Model file for the job. Use its own axes, mm. A direction names the side the tool comes from. Coordinates: 2 decimals unless noted, no trailing zeros. Loops run counter-clockwise (first coordinate to the right, second up) from the corner with the lowest first, then second, coordinate; pieces in that order, holes last. Notation, with made-up numbers: (68, 79) -> (83, 79) arc R12 cw to (83, 95) -> close; hole circle Ø2 at (-37.5, -31.5). An arc over 180 degrees is marked (long way). Use one line per item in the form item = value.
```python
from build123d import *

# Parameters (mm, degrees)
SKETCH1_W           = 150
SKETCH1_H           = 40
BOSS_EXTRUDE1_DEPTH = 10
BOSS_EXTRUDE2_DEPTH = 10
CUT_EXTRUDE1_DEPTH  = 121.208152802
SKETCH8_R           = 3.5
CUT_EXTRUDE2_DEPTH  = 108.935165725
FILLET1_R           = 3


with BuildPart() as part:
    # Sketch1 → Boss-Extrude1 (new body)
    with BuildSketch(Plane(origin=(0, 0, 0), x_dir=(1, 0, 0), z_dir=(0, 1, 0))):
        Rectangle(SKETCH1_W, SKETCH1_H)
    extrude(amount=BOSS_EXTRUDE1_DEPTH)

    # Sketch2 → Boss-Extrude2 (add)
    with BuildSketch(Plane.XY.offset(20)):
        with BuildLine():
            Line((-45, 10), (-5, 10))
            Line((-5, 10), (-5, 65))
            ThreePointArc((-5, 65), (-25, 85), (-45, 65))
            Line((-45, 65), (-45, 10))
        make_face()
    extrude(amount=-BOSS_EXTRUDE2_DEPTH)

    # Sketch6 → CBORE for M6 SBHCS1 (revolve, cut)
    with BuildSketch(Plane(origin=(-25, 65, 10), x_dir=(0, 1, 0), z_dir=(1, 0, 0))):
        Polygon((0, 0), (0, 10), (9.005, 10), (9.005, 5.68), (4.5, 5.68), (4.5, 0), align=None)
    revolve(axis=Axis((-25, 65, 3.65), (0, 0, 1)), mode=Mode.SUBTRACT)

    # Sketch7 → Cut-Extrude1 (cut, through all)
    with BuildSketch(Plane.XY.offset(20)):
        with BuildLine():
            Line((-39.803847577, 3), (-10.196152423, 3))
            ThreePointArc((-10.196152423, 3), (-7.196152423, 2.196152423), (-5, 0))
            Line((-5, 0), (-45, 0))
            ThreePointArc((-45, 0), (-42.803847577, 2.196152423), (-39.803847577, 3))
        make_face()
    extrude(amount=-CUT_EXTRUDE1_DEPTH, mode=Mode.SUBTRACT)

    # Sketch8 → Cut-Extrude2 (cut, through all)
    with BuildSketch(Plane(origin=(0, 10, 0), x_dir=(1, 0, 0), z_dir=(0, 1, 0))):
        with Locations(Location((-55, 0, 0), (0, 0, 270))):
            Circle(SKETCH8_R)
        with Locations(Location((55, 0, 0), (0, 0, 270))):
            Circle(SKETCH8_R)
    extrude(amount=-CUT_EXTRUDE2_DEPTH, mode=Mode.SUBTRACT)

    # Fillet1
    fillet1_edges = [part.edges().sort_by_distance(p)[0] for p in [
        (-75, 10, 0),
        (35, 10, 20),
        (-45, 37.5, 10),
        (-45, 10, 15),
        (-25, 85, 10),
        (-5, 37.5, 10),
        (-60, 10, 20),
        (-25, 10, 10),
        (-5, 10, 15),
        (-45, 37.5, 20),
        (-5, 37.5, 20),
        (-25, 85, 20),
        (75, 10, 0),
        (75, 5, 20),
        (-75, 5, 20),
        (-75, 5, -20),
        (75, 5, -20),
        (0, 10, -20),
    ]]
    fillet(fillet1_edges, radius=FILLET1_R)


solid = part.part
```
Q1. Band-saw the part on A-A, the plane z = 0. Write the cut outline in (x, y), and give its area (3 significant figures).
Result:
outline = (-75, 0) -> (-58.5, 0) -> (-58.5, 10) -> (-72, 10) arc R3 ccw to (-75, 7) -> close; (-51.5, 0) -> (-45, 0) arc R6 cw to (-39.8, 3) -> (-10.2, 3) arc R6 cw to (-5, 0) -> (51.5, 0) -> (51.5, 10) -> (-51.5, 10) -> close; (58.5, 0) -> (75, 0) -> (75, 7) arc R3 ccw to (72, 10) -> (58.5, 10) -> close
area = 1,250 mm2
Q2. Band-saw the part on D-D, the plane y = 29.5. Write the cut outline in (x, z).
Result:
outline = (-45, 13) arc R3 ccw to (-42, 10) -> (-8, 10) arc R3 ccw to (-5, 13) -> (-5, 17) arc R3 ccw to (-8, 20) -> (-42, 20) arc R3 ccw to (-45, 17) -> close
Q3. Wall check: line 1 along X through (y, z) = (4.5, 0); line 2 along X through (y, z) = (65, 12.65); line 3 along Y through (x, z) = (-25, 14.35). Give the ranges that are in metal, low to high.
Result:
line_1 = -75 to -58.5, -51.5 to 51.5, 58.5 to 75
line_2 = -44.98 to -29.5, -20.5 to -5.02
line_3 = 3 to 60.5, 69.5 to 85
Q4. Mould opens along X. For faces 1 (the face through (-59.83, 9.1, 19.14)), 2 (the face through (58.47, 5.07, -0.46)), 3 (the face through (-21, 69, 15.68)), 4 (the face through (75, 3, 0)) say: released by +X, released by -X, zero draft, split by the parting line, or undercut.
Result:
face_1 = zero draft
face_2 = undercut
face_3 = undercut
face_4 = released by +X
Q5. Which spindle directions (+Z, -Z, +X, -X, +Y, -Y) get a long thin tool onto all of the face, cutting with end or side? Do faces 5 (the face through (-5.9, 39.36, 19.14)), 6 (the face through (-25, 48, 10)), 7 (the face through (-44.1, 38.64, 19.14)), 8 (the face through (-25, 3, 0)). Say none if no direction does.
Result:
face_5 = +Z, +X, +Y
face_6 = -Z, +X, -X, +Y
face_7 = +Z, -X, +Y
face_8 = +Z, -Z, -Y
Q6. Pin check, flat tips, straight feed: pin 1 Ø12 at (y, z) = (71.5, 8) entering from -X; pin 2 Ø16 at (x, y) = (-25, 65) entering from +Z; pin 3 Ø2 at (y, z) = (50.5, 15.5) entering from -X. Stop position of each tip, or through.
Result:
pin_1 = -44.8
pin_2 = 15.68
pin_3 = -45
Q7. Band-saw the part on B-B, the plane x = -25. Write the cut outline in (y, z) (3 decimals), and give its area (3 significant figures).
Result:
outline = (3, -20) -> (7, -20) arc R3 ccw to (10, -17) -> (10, 7) arc R3 cw to (13, 10) -> (60.5, 10) -> (60.5, 15.68) -> (55.995, 15.68) -> (55.995, 20) -> (3, 20) -> close; (69.5, 10) -> (82, 10) arc R3 ccw to (85, 13) -> (85, 17) arc R3 ccw to (82, 20) -> (74.005, 20) -> (74.005, 15.68) -> (69.5, 15.68) -> close
area = 897 mm2
Q8. Band-saw the part on C-C, the plane z = -6.5. Write the cut outline in (x, y).
Result:
outline = (-75, 0) -> (-45, 0) arc R6 cw to (-39.8, 3) -> (-10.2, 3) arc R6 cw to (-5, 0) -> (75, 0) -> (75, 7) arc R3 ccw to (72, 10) -> (-72, 10) arc R3 ccw to (-75, 7) -> close
